The drawing under review shows one solid part. Ordinate dimensions are in mm from its lowest x, y, z. Coordinates: 2 decimals unless noted, no trailing zeros. Order: outer loops, then holes, each group sorted by start corner. A loop starts at its lowest first (then second) coordinate and runs counter-clockwise, first axis right, second up. Notation, with made-up numbers: (19.5, 33) - (32.5, 33) arc R31 cw to (32.5, 72) - close; hole circle Ø5 at (66.25, -6). An arc over 180 degrees is marked (long way). Answer in a Markdown table with one row per item.
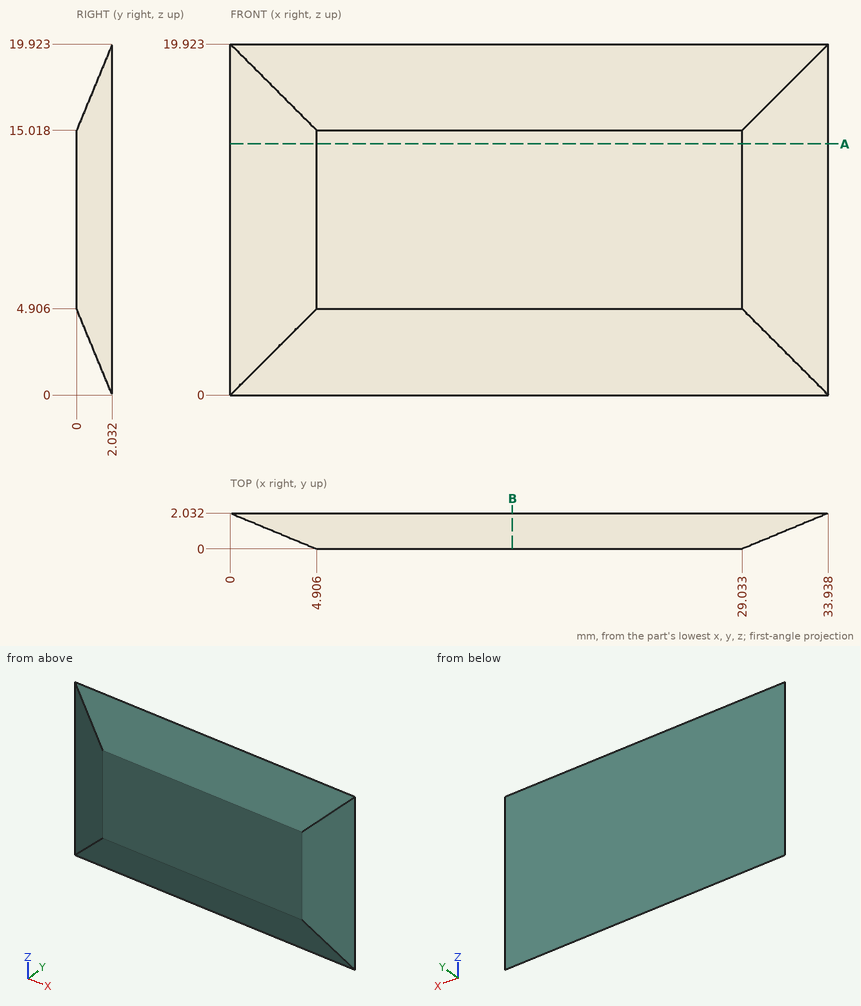
Item 1: Clearance check with a flat-ended pin moving along its axis: pin 1 Ø8 at (x, z) = (16.5, 3) entering from -Y. State where the tip first meets the part, or that it passes through.
Check values:
| item | result |
|---|---|
| pin 1 | y = 0 |
Item 2: We need section B-B, the plane x = 16. Write out the cut boundary in (y, z) (1 decimal).
Check values:
| item | result |
|---|---|
| outline | (0, 4.9) - (2, 0) - (2, 19.9) - (0, 15) - close |
Item 3: We need section A-A, the plane z = 14.25. Write out the cut boundary in (x, y) (1 decimal).
Check values:
| item | result |
|---|---|
| outline | (0, 2) - (4.9, 0) - (29, 0) - (33.9, 2) - close |
Item 4: To check wall thickness, follow line 1 (Z direction, x = 3.5, y = 1.25) (1 decimal); line 2 (Z direction, x = 15.5, y = 1.85) (1 decimal); line 3 (X direction, y = 0.7, z = 6.25) (1 decimal). State the ranges of each line that lie inside material, in increasing order. Write a range as from..to.
Check values:
| item | result |
|---|---|
| line 1 | 1.9..18 |
| line 2 | 0.4..19.5 |
| line 3 | 3.2..30.7 |
